CAD build for the part. Positions are in the model's coordinates, mm. Face numbers are marked on the shaded views. Coordinates: 2 decimals unless noted, no trailing zeros. Order: outer loops, then holes, each group sorted by start corner. A loop starts at its lowest first (then second) coordinate and runs counter-clockwise, first axis right, second up. Notation, with made-up numbers: (20.25, -36.75) - (63.25, -36.75) arc R17 cw to (63.25, -19.75) - close; hole circle Ø3 at (3.5, 35). An arc over 180 degrees is marked (long way). Use one line per item in the form item = value.
```python
from build123d import *

# Parameters (mm, degrees)
SKETCH1_R           = 4
BOSS_EXTRUDE1_DEPTH = 47
SKETCH2_R           = 1.4
CUT_EXTRUDE1_DEPTH  = 10
CUT_EXTRUDE2_START  = -35
SKETCH3_R           = 4
SKETCH3_R_2         = 3.6
CUT_EXTRUDE2_DEPTH  = 15


with BuildPart() as part:
    # Sketch1 → Boss-Extrude1 (new, symmetric)
    with BuildSketch(Plane(origin=(0, 0, 0), x_dir=(1, 0, 0), z_dir=(0, 1, 0))):
        with Locations(Location((0, 0, 0), (0, 0, 270))):
            Circle(SKETCH1_R)
    extrude(amount=BOSS_EXTRUDE1_DEPTH, both=True)

    # Sketch2 → Cut-Extrude1 (cut)
    with BuildSketch(Plane.XZ.offset(47)):
        with Locations(Location((0, 0, 0), (0, 0, 270))):
            Circle(SKETCH2_R)
    cut_extrude1 = extrude(amount=-CUT_EXTRUDE1_DEPTH, mode=Mode.SUBTRACT)

    # Mirror1: Cut-Extrude1 across plane
    add(cut_extrude1.mirror(Plane.ZX), mode=Mode.SUBTRACT)

    # Sketch3 → Cut-Extrude2 (cut)
    with BuildSketch(Plane.XZ.offset(47).offset(CUT_EXTRUDE2_START)):
        with Locations(Location((0, 0, 0), (0, 0, 270))):
            Circle(SKETCH3_R)
        with Locations(Location((0, 0, 0), (0, 0, 270))):
            Circle(SKETCH3_R_2, mode=Mode.SUBTRACT)
    extrude(amount=CUT_EXTRUDE2_DEPTH, mode=Mode.SUBTRACT)


solid = part.part
```
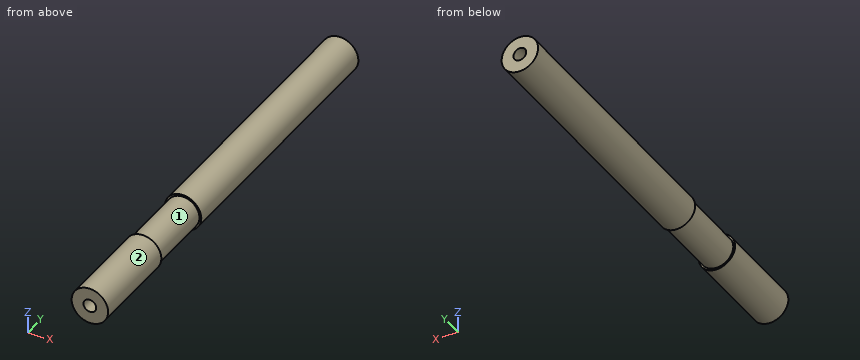
Item 1: Drop flat-ended pins along their axis: pin 1 (1.7 mm diameter, centred on x = 0, z = 0, fed in from +Y); pin 2 (4 mm diameter, centred on y = -27, z = 2.5, fed in from -X); pin 3 (2 mm diameter, centred on x = 0, z = 0, fed in from -Y). Give the stop position or say it passes through.
Derived:
pin_1 = 37
pin_2 = -3.97
pin_3 = -37
Item 2: Cut at A-A, the plane z = 0. Write the cut outline in (x, y).
Derived:
outline = (-4, -47) - (-1.4, -47) - (-1.4, -37) - (1.4, -37) - (1.4, -47) - (4, -47) - (4, -27) - (3.6, -27) - (3.6, -12) - (4, -12) - (4, 47) - (1.4, 47) - (1.4, 37) - (-1.4, 37) - (-1.4, 47) - (-4, 47) - (-4, -12) - (-3.6, -12) - (-3.6, -27) - (-4, -27) - close
Item 3: Cut at D-D, the plane y = 38. Write the cut outline in (x, z), plus the area to 3 significant figures.
Derived:
outline = circle Ø8 at (0, 0); hole circle Ø2.8 at (0, 0)
area = 44.1 mm²
Item 4: Drill centre lines: line 1 (Y direction, x = -3, z = -2.5); line 2 (X direction, y = -44, z = 0); line 3 (Z direction, x = -1.75, y = 12.5). Where is each one in solid material? Low to high. Write a range as [from, to].
Derived:
line_1 = [-47, -27], [-12, 47]
line_2 = [-4, -1.4], [1.4, 4]
line_3 = [-3.6, 3.6]
Item 5: Cut at B-B, the plane x = -2.5. Write the cut outline in (y, z).
Derived:
outline = (-47, -3.12) - (-27, -3.12) - (-27, -2.59) - (-12, -2.59) - (-12, -3.12) - (47, -3.12) - (47, 3.12) - (-12, 3.12) - (-12, 2.59) - (-27, 2.59) - (-27, 3.12) - (-47, 3.12) - close
Item 6: Two-plate mould, pull along Y, no slides. Class the marked faces 1 and 2: +Y half, -Y half, draft (parallel to the pull), parting line (faces both ways), or undercut.
Derived:
face_1 = undercut
face_2 = draft
Item 7: Cut at C-C, the plane y = 21.5. Write the cut outline in (x, z), plus the area to 3 significant figures.
Derived:
outline = circle Ø8 at (0, 0)
area = 50.3 mm²
